from build123d import *

# Parameters (mm, degrees)
CHAMFER1_SIZE      = 0.79375
CHAMFER2_SIZE      = 0.36115625
CHAMFER3_SIZE      = 0.2032
CUT_EXTRUDE2_DEPTH = 2.778125


with BuildPart() as part:
    # Sketch1 → Revolve1 (revolve)
    with BuildSketch(Plane(origin=(0, 0, 0), x_dir=(0, 0, -1), z_dir=(1, 0, 0))):
        Polygon((0, 5.55625), (5.55625, 5.55625), (5.55625, 3.96875), (59.53125, 3.96875), (59.53125, 3.175), (70.64375, 3.175), (70.64375, 0), (0, 0), align=None)
    revolve(axis=Axis((0, 0, -70.64375), (0, 0, 1)))

    # Sketch5 → Cut-Revolve1 (revolve, cut)
    with BuildSketch(Plane(origin=(0, 0, 0), x_dir=(0, 0, -1), z_dir=(1, 0, 0))):
        with BuildLine():
            Line((59.53125, 3.96875), (63.5889, 3.96875))
            Line((63.5889, 3.96875), (62.07125, 2.4511))
            Line((62.07125, 2.4511), (60.25515, 2.4511))
            ThreePointArc((60.25515, 2.4511), (59.743275401, 2.663125401), (59.53125, 3.175))
            Line((59.53125, 3.175), (59.53125, 3.96875))
        make_face()
    revolve(axis=Axis((0, 0, -70.64375), (0, 0, 1)), mode=Mode.SUBTRACT)

    # Chamfer1
    chamfer1_edges = [part.edges().sort_by_distance(p)[0] for p in [
        (0, -3.175, -70.64375),
    ]]
    chamfer(chamfer1_edges, length=CHAMFER1_SIZE)

    # Chamfer2
    chamfer2_edges = [part.edges().sort_by_distance(p)[0] for p in [
        (0, -5.55625, 0),
    ]]
    chamfer(chamfer2_edges, length=CHAMFER2_SIZE)

    # Chamfer3
    chamfer3_edges = [part.edges().sort_by_distance(p)[0] for p in [
        (0, -3.96875, -59.53125),
    ]]
    chamfer(chamfer3_edges, length=CHAMFER3_SIZE)

    # Sketch8 → Cut-Extrude2 (cut)
    with BuildSketch(Plane.XY):
        Polygon((1.984375, 1.14567944), (0, 2.291358881), (-1.984375, 1.14567944), (-1.984375, -1.14567944), (0, -2.291358881), (1.984375, -1.14567944), align=None)
    extrude(amount=-CUT_EXTRUDE2_DEPTH, mode=Mode.SUBTRACT)

    # Cut-Extrude4 cone 1 section (through the dimple's axis) → Cut-Extrude4 (revolve, cut)
    with BuildSketch(Plane(origin=(0, 0, 0), x_dir=(0, -1, 0), z_dir=(1, 0, 0))):
        Polygon((0, 0), (2.291358881, 0), (0, 2.291358881), align=None)
    revolve(axis=Axis((0, 0, 0), (0, 0, -1)), mode=Mode.SUBTRACT)


solid = part.part
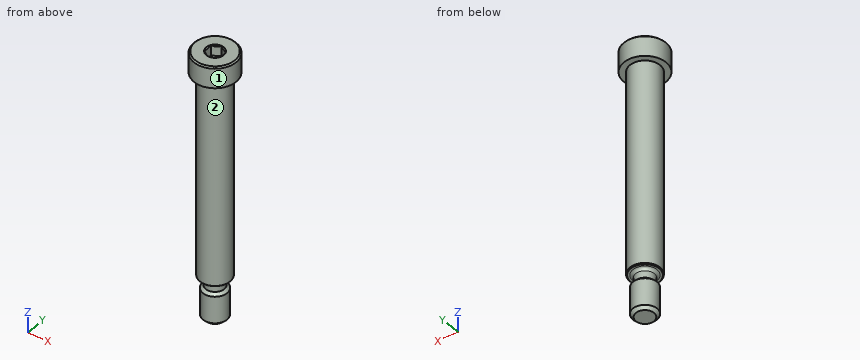
The listing builds one solid part. Answer for the finished solid, in the listing's coordinates (mm). Face numbers are marked on the shaded views. A direction names the side the tool comes from. Give positions to 0.01 mm unless a question says otherwise; leave off trailing zeros. Write each loop counter-clockwise with the first axis right and the second up, starting at its lowest first coordinate (ties: lowest second). Pieces come first, ordered by that corner, then holes. Notation, with made-up numbers: (63.5, 85.5) -> (102.5, 85.5) arc R19 ccw to (102.5, 90.5) -> close; hole circle Ø11 at (69, 66.5). An arc over 180 degrees is marked (long way). One line per question, with ' | ' between items. Start each with the question number.
1. Find the intervals of material crossed by probe 1 along Y at (x, z) = (3.25, -47); probe 2 along Z at (x, y) = (-0.5, 4.25); probe 3 along Y at (x, z) = (-0.25, -29), in increasing order.
2. Given pin 1 Ø3 at (x, z) = (0.5, -54) entering from -Y; pin 2 Ø5 at (x, y) = (4, 3.5) entering from -Z; pin 3 Ø6 at (x, z) = (3.5, -31.5) entering from +Y, each flat-ended and moving along its own axis, determine where each tip first touches the part or whether it passes through.
3. Section C-C (z = -34) is taken. Determine the outline of the cut face in (x, y), plus the area to 3 significant figures.
4. For the marked faces 1 and 2, determine the directions among +Z, -Z, +X, -X, +Y, -Y from which every point of the face is accessible in a straight line to the end or side of a thin tool.
5. Section B-B (z = -4) is taken. Determine the outline of the cut face in (x, y), plus the area to 3 significant figures.
Response values:
1) probe 1: -2.28 to 2.28 | probe 2: -5.56 to 0 | probe 3: -3.96 to 3.96
2) pin 1: y = -3.97 | pin 2: z = -70.21 | pin 3: y = 3.94
3) outline: circle Ø7.94 at (0, 0) | area: 49.5 mm2
4) face 1: +Z, -Z | face 2: -Z
5) outline: circle Ø11.11 at (0, 0) | area: 97.0 mm2
